from build123d import *

# Parameters (mm, degrees)
SKETCH2_R           = 0.775
SKETCH2_R_2         = 4.875
BOSS_EXTRUDE1_DEPTH = 2.5


with BuildPart() as part:
    # Sketch2 → Boss-Extrude1 (new body)
    with BuildSketch(Plane(origin=(0, 0, 0), x_dir=(1, 0, 0), z_dir=(0, 1, 0))):
        with BuildLine():
            Line((-57.445626465, 40), (-120, 40))
            Line((-120, 40), (-120, -40))
            Line((-120, -40), (-57.445626465, -40))
            ThreePointArc((-57.445626465, -40), (0, -70), (57.445626465, -40))
            Line((57.445626465, -40), (120, -40))
            Line((120, -40), (120, 40))
            Line((120, 40), (57.445626465, 40))
            ThreePointArc((57.445626465, 40), (0, 70), (-57.445626465, 40))
        make_face()
        with Locations((0, 24)):
            Circle(SKETCH2_R, mode=Mode.SUBTRACT)
        with Locations((0, -24)):
            Circle(SKETCH2_R, mode=Mode.SUBTRACT)
        Circle(SKETCH2_R_2, mode=Mode.SUBTRACT)
    extrude(amount=BOSS_EXTRUDE1_DEPTH)


solid = part.part
Input: part model. Units: mm. Frame: model coordinates. Coordinates: 2 decimals unless noted, no trailing zeros. Write each loop counter-clockwise with the first axis right and the second up, starting at its lowest first coordinate (ties: lowest second). Pieces come first, ordered by that corner, then holes. Notation, with made-up numbers: M 57,65 L 81,65 A8 cw 81,70 Z; hole C 22,-19.5 d1. An arc over 180 degrees is marked long. Answer as a JSON object with one key per item and string values. Group by question number.
(1) Ray query, line 1 along Z through (x, y) = (0, 1.7) (3 decimals); line 2 along X through (y, z) = (1.5, 24) (3 decimals); line 3 along X through (y, z) = (1, 0) (3 decimals). Return the intervals inside material, ascending. Write a range as [from, to].
(2) Mould query, pull axis Z, two halves, no side actions, for faces 1 (the face through (-0.635, 1.232, -4.834)), 2 (the face through (0.943, 1.232, -69.994)), 3 (the face through (-0.943, 1.232, 69.994)). Classes: pulls with the +Z half, pulls with the -Z half, needs draft (parallel to the pull), parting line crosses it, or undercut.
(3) Section C-C on x = -66.5. Output: boundary loops of the cut face in (y, z), plus the area to 3 significant figures.
(4) Section D-D on z = -42.5. Output: boundary loops of the cut face in (x, y), plus the area to 3 significant figures.
(5) Section A-A on z = 0. Output: boundary loops of the cut face in (x, y) (3 decimals), plus the area to 3 significant figures.
(6) Contact query for flat-ended pins moving along their axis: P1, Ø1.2, axis at x = -100.5, y = 1, coming from the +Z side; P2, Ø1, axis at y = 0.5, z = 49.5, coming from the +X side; P3, Ø1.4, axis at x = 0, z = 24, coming from the -Y side (3 decimals). Output: stop coordinate, or through.
(7) Section B-B on y = 1.75. Output: boundary loops of the cut face in (x, z) (3 decimals).
Result set:
{
 "1": {"line 1": "z = [-70, -24.775], [-23.225, -4.875], [4.875, 23.225], [24.775, 70]", "line 2": "x = [-120, -0.775], [0.775, 120]", "line 3": "x = [-120, -4.875], [4.875, 120]"},
 "2": {"face 1": "undercut", "face 2": "pulls with the -Z half", "face 3": "pulls with the +Z half"},
 "3": {"outline": "M 0,-40 L 2.5,-40 L 2.5,40 L 0,40 Z", "area": "200 mm2"},
 "4": {"outline": "M -55.62,0 L 55.62,0 L 55.62,2.5 L -55.62,2.5 Z", "area": "278 mm2"},
 "5": {"outline": "M -120,0 L -4.875,0 L -4.875,2.5 L -120,2.5 Z; M 4.875,0 L 120,0 L 120,2.5 L 4.875,2.5 Z", "area": "576 mm2"},
 "6": {"P1": "stops at z = 40", "P2": "stops at x = 49.99", "P3": "passes through"},
 "7": {"outline": "M -120,-40 L -57.446,-40 A70 ccw 57.446,-40 L 120,-40 L 120,40 L 57.446,40 A70 ccw -57.446,40 L -120,40 Z; hole C 0,0 d9.75; hole C 0,-24 d1.55; hole C 0,24 d1.55"}
}
